Source: CAD feature listing. Evaluate the final solid. Frame: model axes, mm. A direction names the side the tool comes from. Coordinates: 2 decimals unless noted, no trailing zeros. Loops run counter-clockwise (first coordinate to the right, second up) from the corner with the lowest first, then second, coordinate; pieces in that order, holes last. Notation, with made-up numbers: (-15.75, 31.5) -> (42.25, 31.5) arc R7 cw to (42.25, 38.5) -> close; hole circle Ø3 at (77, 29.25). An arc over 180 degrees is marked (long way). Answer as a JSON object with one key per item and string values. Group by question number.
Autodesk Inventor part; units mm, degrees
ref_plane "YZ Plane" through (0, 0, 0) normal (1, 0, 0) x (0, 1, 0)
ref_plane "XZ Plane" through (0, 0, 0) normal (0, 1, 0) x (-1, 0, 0)
ref_plane "XY Plane" through (0, 0, 0) normal (0, 0, 1) x (1, 0, 0)
sketch "Sketch1" plane through (0, 0, 0) normal (0, 1, 0) x (-1, 0, 0)
  line L0 (3.1454, 6.687) -> (-3.2046, 6.687)
  line L1 (-3.2046, 6.687) -> (-3.2046, -37.763)
  line L2 (-3.2046, -37.763) -> (3.1454, -37.763)
  line L3 (3.1454, -37.763) -> (3.1454, 6.687)
  point P0 (0, 0)
  dimension "d0" = 6.35
  dimension "d1" = 44.45
extrude "Extrusion1" add sketch "Sketch1" along normal blind 25.4
sketch "Sketch2" plane through (3.2046, 0, 6.687) normal (1, 0, 0) x (0, 0, -1)
  line L0 (0, 0) -> (0, 25.4)
  point P0 (6.687, 0)
  point P1 (19.05, 12.4335)
  dimension "d4" = 19.05
hole "Hole1" at (3.2046, 12.4335, -12.363) direction (-1, 0, 0) diameter 6.7564 end through all counterbore diameter 12.7 counterbore depth 3.175
sketch "Sketch4" plane through (-3.1454, 0, -37.763) normal (-1, 0, 0) x (0, 0, 1)
  line L0 (44.45, 0) -> (44.45, 25.4)
  point P0 (37.763, 0)
  point P1 (14.7574, 12.7)
  dimension "d20" = 29.6926
hole "Hole3" at (-3.1454, 12.7, -23.0056) direction (1, 0, 0) diameter 2.4867 end through all
sketch "Sketch5" plane through (-3.1454, 0, -37.763) normal (-1, 0, 0) x (0, 0, 1)
  line L0 (44.45, 0) -> (44.45, 25.4)
  line L1 (0, 25.4) -> (44.45, 25.4)
  point P0 (37.763, 0)
  point P1 (36.9824, 12.7)
  dimension "d28" = 7.4676
  dimension "d36" = 12.7
hole "Hole4" at (-3.1454, 12.7, -0.7806) direction (1, 0, 0) diameter 2.4867 end through all
equation "\"d22\" = d20"
equation "\"d30\" = d28"
properties part number "Zero Dead Space Electronic needle valve holder Newst"
1. Section query C-C on y = 17.5. Return loops of the section in (x, z), then the cut area to 3 significant figures.
2. Reachability of faces 4 (the face through (1.595, 8.142, -7.683)), 5 (the face through (0, 25.4, -15)) from +Z, -Z, +X, -X, +Y, -Y: full face, straight path, thin tool, end or side. Return the list, or none.
3. Section query B-B on x = 2. Return loops of the section in (y, z).
4. Pin query (flat end, axial travel): pin 1 Ø1.5 at (y, z) = (12.7, -0.78) entering from -X. Return the tip coordinate at first contact, or that it passes through.
5. Mould query, pull axis Y, two halves, no side actions, for faces 1 (the face through (3.205, 13, -20)), 2 (the face through (0.07, 11.86, -1.7)), 3 (the face through (0, 0, -15)). Classes: pulls with the +Y half, pulls with the -Y half, needs draft (parallel to the pull), parting line crosses it, or undercut.
6. Section query D-D on z = -10. Return loops of the section in (x, y).
7. Ray query, L1, parallel to Z at x = -1.5, y = 12.7; L2, parallel to Y at x = 3, z = -23; L3, parallel to Y at x = 1.75, z = -7. Return the intervals inside material, ascending.
8. Section query A-A on z = 0. Return loops of the section in (x, y), then the cut area to 3 significant figures.
Solved:
{
 "1": {"outline": "(-3.15, -37.76) -> (3.2, -37.76) -> (3.2, -16.19) -> (0.03, -16.19) -> (0.03, -8.54) -> (3.2, -8.54) -> (3.2, 6.69) -> (-3.15, 6.69) -> close", "area": "258 mm^2"},
 "2": {"face 4": "+X", "face 5": "+Z, -Z, +X, -X, +Y"},
 "3": {"outline": "(0, -37.76) -> (25.4, -37.76) -> (25.4, 6.69) -> (0, 6.69) -> close; hole circle Ø12.7 at (12.43, -12.36); hole circle Ø2.49 at (12.7, -23.01); hole circle Ø2.49 at (12.7, -0.78)"},
 "4": {"pin 1": "through"},
 "5": {"face 1": "needs draft", "face 2": "undercut", "face 3": "pulls with the -Y half"},
 "6": {"outline": "(-3.15, 0) -> (3.2, 0) -> (3.2, 6.54) -> (0.03, 6.54) -> (0.03, 10.02) -> (-3.15, 10.02) -> close; (-3.15, 14.85) -> (0.03, 14.85) -> (0.03, 18.33) -> (3.2, 18.33) -> (3.2, 25.4) -> (-3.15, 25.4) -> close"},
 "7": {"L1": "-37.76 to -24.25, -21.76 to -15.73, -9 to -2.02, 0.46 to 6.69", "L2": "0 to 11.46, 13.94 to 25.4", "L3": "0 to 9.03, 15.83 to 25.4"},
 "8": {"outline": "(-3.15, 0) -> (3.2, 0) -> (3.2, 11.73) -> (-3.15, 11.73) -> close; (-3.15, 13.67) -> (3.2, 13.67) -> (3.2, 25.4) -> (-3.15, 25.4) -> close", "area": "149 mm^2"}
}
